```python
from build123d import *

# Parameters (mm, degrees)
RESSALTO_EXTRUS_O2_DEPTH   = 20
ESBO_O2_R                  = 1.6
CORTE_EXTRUS_O1_DEPTH      = 2.5
CORTE_EXTRUS_O2_REACH      = 46.218
CORTE_EXTRUS_O2_END_RADIUS = 55
ESBO_O3_R                  = 3.1


with BuildPart() as part:
    # Esboço1 → Ressalto-extrusão2 (new body)
    with BuildSketch(Plane.XY):
        with BuildLine():
            Line((-15, -45.899794856), (-15, -17.899794856))
            Line((-15, -17.899794856), (15, -17.899794856))
            Line((15, -17.899794856), (15, -45.899794856))
            Line((15, -45.899794856), (25, -45.899794856))
            Line((25, -45.899794856), (25, -48.989794856))
            ThreePointArc((25, -48.989794856), (0, -55), (-25, -48.989794856))
            Line((-25, -48.989794856), (-25, -45.899794856))
            Line((-25, -45.899794856), (-15, -45.899794856))
        make_face()
    extrude(amount=RESSALTO_EXTRUS_O2_DEPTH)

    # Esboço2 → Corte-extrusão1 (cut)
    with BuildSketch(Plane(origin=(0, -45.899794856, 0), x_dir=(1, 0, 0), z_dir=(0, 1, 0))):
        with Locations(Location((-21, -10, 0), (0, 0, 270))):
            Circle(ESBO_O2_R)
        with Locations(Location((21, -10, 0), (0, 0, 270))):
            Circle(ESBO_O2_R)
    extrude(amount=-CORTE_EXTRUS_O1_DEPTH, mode=Mode.SUBTRACT)

    # Corte-extrusão2: up to this cylinder (the profile starts inside it)
    corte_extrus_o2_end = Plane(origin=(0, 0, 10), z_dir=(0, 0, -1)) * Cylinder(CORTE_EXTRUS_O2_END_RADIUS, 203.436, mode=Mode.PRIVATE)
    # Esboço3 → Corte-extrusão2 (cut, up to the surface)
    with BuildSketch(Plane(origin=(0, -48.399794856, 0), x_dir=(1, 0, 0), z_dir=(0, 1, 0)), mode=Mode.PRIVATE) as corte_extrus_o2_sk1:
        with Locations(Location((-21, -10, 0), (0, 0, 270))):
            Circle(ESBO_O3_R)
    corte_extrus_o2_tool1 = extrude(corte_extrus_o2_sk1.sketch, amount=-CORTE_EXTRUS_O2_REACH, mode=Mode.PRIVATE) & corte_extrus_o2_end
    add(corte_extrus_o2_tool1.solids().sort_by_distance((-21, -48.399795, 10))[0], mode=Mode.SUBTRACT)
    # Esboço3 → Corte-extrusão2 (cut, up to the surface)
    with BuildSketch(Plane(origin=(0, -48.399794856, 0), x_dir=(1, 0, 0), z_dir=(0, 1, 0)), mode=Mode.PRIVATE) as corte_extrus_o2_sk2:
        with Locations(Location((21, -10, 0), (0, 0, 270))):
            Circle(ESBO_O3_R)
    corte_extrus_o2_tool2 = extrude(corte_extrus_o2_sk2.sketch, amount=-CORTE_EXTRUS_O2_REACH, mode=Mode.PRIVATE) & corte_extrus_o2_end
    add(corte_extrus_o2_tool2.solids().sort_by_distance((21, -48.399795, 10))[0], mode=Mode.SUBTRACT)


solid = part.part
```
The model under review builds one solid part; all positions refer to its coordinate system, in mm. A direction names the side the tool comes from. Give positions to 0.01 mm unless a question says otherwise; leave off trailing zeros. Write each loop counter-clockwise with the first axis right and the second up, starting at its lowest first coordinate (ties: lowest second). Pieces come first, ordered by that corner, then holes.
(1) Consider section A-A, the plane x = 21. Give the boundary of the cut face in (y, z), and give its area (3 significant figures).
(2) Tool access review of faces 5 (the flat face through (0, -36, 0)), 6 (the flat face through (15, -32, 10)), 7 (the flat face through (-22.3, -48.4, 11.3)), 8 (the flat face through (-15, -32, 10)): name each direction out of +Z, -Z, +X, -X, +Y, -Y from which nothing blocks a thin tool from reaching the whole face with its end or side.
(3) Consider section C-C, the plane z = 10. Give the boundary of the cut face in (x, y), and give its area (3 significant figures).
(4) The part is to be moulded in two halves that separate along X. For faces 1 (the flat face through (25, -47, 10)), 2 (the flat face through (-25, -47, 10)), 3 (the flat face through (19, -45.9, 10)), 4 (the cylindrical face through (17.974, -49.777, 9.328)), say which applies: released by +X, released by -X, zero draft, split by the parting line, or undercut.
(5) Consider section D-D, the plane y = -26. Give the boundary of the cut face in (x, z), and give its area (3 significant figures).
(6) For P1, Ø4, axis at y = -37, z = 10, coming from the -X side; P2, Ø5, axis at x = -21, z = 9.5, coming from the +Y side; P3, Ø1.9, axis at x = -21.5, z = 10, coming from the -Y side; P4, Ø7, axis at x = -21, z = 10, coming from the -Y side, all flat-tipped, find the tip position at first contact; note any pin that passes through.
(7) Consider section B-B, the plane z = 15.25. Give the boundary of the cut face in (x, y).
(8) To check wall thickness, follow L1, parallel to X at y = -46.9, z = 10; L2, parallel to Z at x = -21, y = -50.35; L3, parallel to X at y = -23.5, z = 12. State the ranges of each line that lie inside material, in increasing order.
Returned:
1. outline: (-50.83, 0) - (-45.9, 0) - (-45.9, 8.4) - (-48.4, 8.4) - (-48.4, 6.9) - (-50.83, 6.9) - close; (-50.83, 13.1) - (-48.4, 13.1) - (-48.4, 11.6) - (-45.9, 11.6) - (-45.9, 20) - (-50.83, 20) - close
1. area: 75.6 mm2
2. face 5: -Z, +X, -X, +Y, -Y
2. face 6: +Z, -Z, +X, +Y
2. face 7: -Y
2. face 8: +Z, -Z, -X, +Y
3. outline: (-25, -48.99) arc R55 ccw to (-24.1, -49.44) - (-24.1, -48.4) - (-22.6, -48.4) - (-22.6, -45.9) - (-25, -45.9) - close; (-19.4, -48.4) - (-17.9, -48.4) - (-17.9, -52.01) arc R55 ccw to (17.9, -52.01) - (17.9, -48.4) - (19.4, -48.4) - (19.4, -45.9) - (15, -45.9) - (15, -17.9) - (-15, -17.9) - (-15, -45.9) - (-19.4, -45.9) - close; (22.6, -48.4) - (24.1, -48.4) - (24.1, -49.44) arc R55 ccw to (25, -48.99) - (25, -45.9) - (22.6, -45.9) - close
3. area: 1,150 mm2
4. face 1: released by +X
4. face 2: released by -X
4. face 3: zero draft
4. face 4: undercut
5. outline: (-15, 0) - (15, 0) - (15, 20) - (-15, 20) - close
5. area: 600 mm2
6. P1: stops at x = -15
6. P2: stops at y = -45.9
6. P3: passes through
6. P4: stops at y = -52.14
7. outline: (-25, -48.99) arc R55 ccw to (25, -48.99) - (25, -45.9) - (15, -45.9) - (15, -17.9) - (-15, -17.9) - (-15, -45.9) - (-25, -45.9) - close
8. L1: x = -25 to -22.6, -19.4 to 19.4, 22.6 to 25
8. L2: z = 0 to 6.9, 13.1 to 20
8. L3: x = -15 to 15
